Input: part model. Units: mm. Frame: model coordinates. A direction names the side the tool comes from. Give positions to 0.01 mm unless a question says otherwise; leave off trailing zeros. Write each loop counter-clockwise with the first axis right and the second up, starting at its lowest first coordinate (ties: lowest second). Pieces come first, ordered by that corner, then holes. Notation, with made-up numbers: (-19.5, 44) -> (-10.5, 44) arc R23 cw to (-10.5, 76) -> close; hole circle Ø3 at (-1, 38.25). An arc over 180 degrees is marked (long way). Return JSON: item names as keys, results as strings. Group by question number.
Item 1: Line query: line 1 (X direction, y = 0, z = 0.25); line 2 (Z direction, x = 9, y = 3.75); line 3 (X direction, y = 0, z = 1.3). Output: solid intervals per line, ascending. Write a range as [from, to].
Item 2: Pin query (flat end, axial travel): P1, Ø5, axis at y = -3, z = -9.5, coming from the +X side; P2, Ø6, axis at x = 14, y = 0, coming from the +Z side; P3, Ø8, axis at x = -10.5, y = 7.5, coming from the -Z side; P4, Ø11, axis at y = -0.5, z = 7, coming from the +X side. Return the tip coordinate at first contact, or that it passes through.
Item 3: Set-up query: faces 1 (the face through (7, 0, -2.5)), 2 (the face through (2, -12.5, 0)), 3 (the face through (0, 0, 6)). Return all of +Z, -Z, +X, -X, +Y, -Y with unobstructed straight access to the full face (end or side cutting, diameter ignored); none if empty.
Item 4: Section B-B, the plane x = 14. Return loops of the section in (y, z), then the cut area to 3 significant figures.
Item 5: Section A-A, the plane y = 0. Return loops of the section in (x, z).
Item 6: Section D-D, the plane x = 2. Return loops of the section in (y, z), then the cut area to 3 significant figures.
Item 7: Mould query, pull axis X, two halves, no side actions, for faces 4 (the face through (0, 0, -6)), 5 (the face through (11.56, 0.54, -0.04)), 6 (the face through (7, 0, 2.5)). Classes: released by +X, released by -X, zero draft, split by the parting line, or undercut.
from build123d import *

# Parameters (mm, degrees)
SKETCH1_R               = 12.5
BOSS_EXTRUDE1_DEPTH     = 27
SKETCH6_W               = 5
SKETCH6_H               = 25
BOSS_EXTRUDE3_DEPTH     = 4.6
BOSS_EXTRUDE4_DEPTH     = 5
CUT_EXTRUDE1_DEPTH      = 34.320414163
CUT_EXTRUDE1_DEPTH_BACK = 34.320414163
SKETCH10_R              = 2.5
REVOLVE1_ANGLE          = 180


with BuildPart() as part:
    # Sketch1 → Boss-Extrude1 (new body)
    with BuildSketch(Plane(origin=(0, 0, 0), x_dir=(0, 0, -1), z_dir=(1, 0, 0))):
        Circle(SKETCH1_R)
    extrude(amount=-BOSS_EXTRUDE1_DEPTH)

    # Sketch6 → Boss-Extrude3 (add)
    with BuildSketch(Plane(origin=(0, 0, 0), x_dir=(0, 0, -1), z_dir=(1, 0, 0))):
        Rectangle(SKETCH6_W, SKETCH6_H)
    extrude(amount=BOSS_EXTRUDE3_DEPTH)

    # Sketch8 → Boss-Extrude4 (add)
    with BuildSketch(Plane.XY.offset(2.5)):
        with BuildLine():
            Line((4.6, 12.5), (4.6, -12.5))
            ThreePointArc((4.6, -12.5), (17.1, 0), (4.6, 12.5))
        make_face()
    extrude(amount=-BOSS_EXTRUDE4_DEPTH)

    # Sketch10 → Cut-Extrude1 (cut, two sides: drawn at the far end of the back side and taken through both)
    with BuildSketch(Plane.XY.offset(2.5).offset(-CUT_EXTRUDE1_DEPTH_BACK)):
        with Locations(Location((14, 0, 0), (0, 0, 270))):
            Circle(SKETCH10_R)
    extrude(amount=CUT_EXTRUDE1_DEPTH + CUT_EXTRUDE1_DEPTH_BACK, mode=Mode.SUBTRACT)

    # Sketch11 → Revolve1 (revolve)
    with BuildSketch(Plane.ZY.offset(27)):
        with BuildLine():
            Line((0, 12.5), (0, -12.5))
            ThreePointArc((0, -12.5), (12.5, 0), (0, 12.5))
        make_face()
    revolve(axis=Axis((-27, 12.5, 0), (0, -1, 0)), revolution_arc=REVOLVE1_ANGLE)


solid = part.part
Answer below:
{
 "1": {"line 1": "x = [-39.5, 11.5], [16.5, 17.1]", "line 2": "z = [-2.5, 2.5]", "line 3": "x = [-39.43, 11.5], [16.5, 17.1]"},
 "2": {"P1": "stops at x = 0", "P2": "stops at z = 2.5", "P3": "stops at z = -12", "P4": "stops at x = 17.1"},
 "3": {"face 1": "-Z, +X, +Y, -Y", "face 2": "+Z, -Z, +X, -X, -Y", "face 3": "+Z, +X, +Y, -Y"},
 "4": {"outline": "(-8.24, -2.5) -> (-2.5, -2.5) -> (-2.5, 2.5) -> (-8.24, 2.5) -> close; (2.5, -2.5) -> (8.24, -2.5) -> (8.24, 2.5) -> (2.5, 2.5) -> close", "area": "57.4 mm2"},
 "5": {"outline": "(-27, -12.5) -> (0, -12.5) -> (0, -2.5) -> (11.5, -2.5) -> (11.5, 2.5) -> (0, 2.5) -> (0, 12.5) -> (-27, 12.5) arc R12.5 ccw to start; (16.5, -2.5) -> (17.1, -2.5) -> (17.1, 2.5) -> (16.5, 2.5) -> close"},
 "6": {"outline": "(-12.5, -2.5) -> (12.5, -2.5) -> (12.5, 2.5) -> (-12.5, 2.5) -> close", "area": "125 mm2"},
 "7": {"face 4": "released by +X", "face 5": "undercut", "face 6": "zero draft"}
}
